For this review, take the finished solid that the model builds, in its own axes (mm). Round coordinates to 2 decimals unless told otherwise and drop trailing zeros. Order: outer loops, then holes, each group sorted by start corner. A loop starts at its lowest first (then second) coordinate and runs counter-clockwise, first axis right, second up. Notation, with made-up numbers: (68, -33.75) - (78, -33.75) arc R20 ccw to (78, -25.75) - close; hole circle Ø10 at (21.25, 70). An arc over 180 degrees is marked (long way). One line per item, written item: value.
Autodesk Inventor part; units mm, degrees
ref_plane "YZ Plane" through (0, 0, 0) normal (1, 0, 0) x (0, 1, 0)
ref_plane "XZ Plane" through (0, 0, 0) normal (0, 1, 0) x (-1, 0, 0)
ref_plane "XY Plane" through (0, 0, 0) normal (0, 0, 1) x (1, 0, 0)
sketch "Sketch1" plane through (0, 0, 0) normal (1, 0, 0) x (0, 1, 0)
  line L0 (3.175, 0) -> (-3.175, 0) construction
  line L1 (3.175, 1.5875) -> (-3.175, 1.5875) construction
  line L2 (-3.175, -1.5875) -> (3.175, -1.5875) construction
  arc A0 (3.175, -1.5875) -> (3.175, 1.5875) centre (3.175, 0) ccw construction
  arc A1 (-3.175, 1.5875) -> (-3.175, -1.5875) centre (-3.175, 0) ccw construction
  circle A2 centre (3.175, -12.7) radius 1.7526
  circle A3 centre (-3.175, -7.9375) radius 1.7526
  line L3 (3.175, -1.8415) -> (-3.175, -1.8415)
  arc A4 (-3.175, 1.8415) -> (-3.175, -1.8415) centre (-3.175, 0) ccw
  line L4 (-3.175, 1.8415) -> (3.175, 1.8415)
  arc A5 (3.175, -1.8415) -> (3.175, 1.8415) centre (3.175, 0) ccw
  arc A6 (1.27, -15.24) -> (6.35, -12.7) centre (3.175, -12.7) ccw
  arc A7 (-6.35, -7.9375) -> (-5.08, -10.4775) centre (-3.175, -7.9375) ccw
  line L5 (-5.08, -10.4775) -> (1.27, -15.24)
  line L6 (6.35, -12.7) -> (6.35, 0)
  line L7 (-6.35, -7.9375) -> (-6.35, 0)
  circle A8 centre (3.175, 12.7) radius 1.7526
  circle A9 centre (-3.175, 7.9375) radius 1.7526
  arc A10 (6.35, 12.7) -> (1.27, 15.24) centre (3.175, 12.7) ccw
  arc A11 (-5.08, 10.4775) -> (-6.35, 7.9375) centre (-3.175, 7.9375) ccw
  line L8 (-5.08, 10.4775) -> (1.27, 15.24)
  line L9 (6.35, 12.7) -> (6.35, 0)
  line L10 (-6.35, 7.9375) -> (-6.35, 0)
  point P0 (0, 0)
  dimension "d0" = 3.175
  dimension "d1" = 3.175
  dimension "d4" = 3.5052
  dimension "d5" = 12.7
  dimension "d6" = 3.175
  dimension "d7" = 3.5052
  dimension "d8" = 3.175
  dimension "d9" = 4.7625
  dimension "d10" = 0.254
  dimension "d11" = 6.35
  dimension "d12" = 6.35
extrude "Extrusion1" add sketch "Sketch1" along normal blind 1.5875
properties part number "Pin Cap - Slot" material "Aluminum 6061"
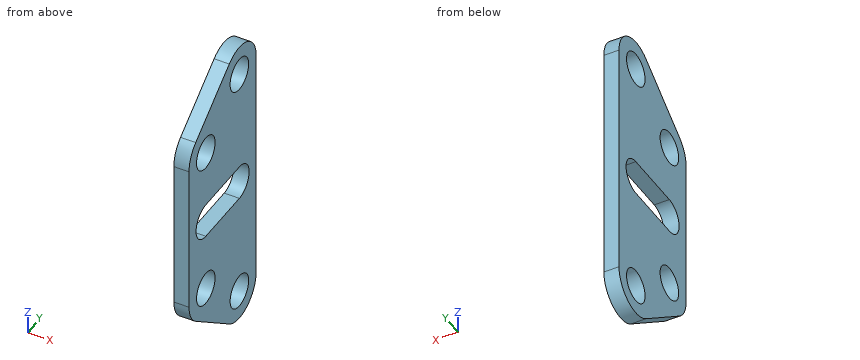
Item 1: Take a section at A-A (x = 0.85). Count the separate pieces of the cut face and the enclosed holes in it, plus the area to 3 significant figures.
Returned:
separate pieces: 1
enclosed holes: 5
area: 272 mm^2
Item 2: Take a section at D-D (z = 10). Write out the cut boundary in (x, y).
Returned:
outline: (0, -5.59) - (1.59, -5.59) - (1.59, 6.35) - (0, 6.35) - close
Item 3: For P1, Ø0.8, axis at x = 0.5, y = -1, coming from the +Z side; P2, Ø0.8, axis at x = 1, y = -0.5, coming from the -Z side, all flat-tipped, find the tip position at first contact; note any pin that passes through.
Returned:
P1: z = 13.84
P2: z = -14.21
Item 4: Take a section at C-C (y = 0.5). Write out the cut boundary in (x, z).
Returned:
outline: (0, -14.66) - (1.59, -14.66) - (1.59, -1.84) - (0, -1.84) - close; (0, 1.84) - (1.59, 1.84) - (1.59, 14.66) - (0, 14.66) - close
Item 5: Take a section at B-B (z = 0). Write out the cut boundary in (x, y).
Returned:
outline: (0, -6.35) - (1.59, -6.35) - (1.59, -5.02) - (0, -5.02) - close; (0, 5.02) - (1.59, 5.02) - (1.59, 6.35) - (0, 6.35) - close
Item 6: Wall thickness on line 1 (Z direction, x = 0.3, y = 4.75); line 2 (Z direction, x = 1, y = 4.25); line 3 (Z direction, x = 0.3, y = -0.25): over which ranges is each line inside the solid? List them lowest first.
Returned:
line 1: -15.46 to -13.47, -11.93 to -0.95, 0.95 to 11.93, 13.47 to 15.46
line 2: -15.69 to -14.08, -11.32 to -1.5, 1.5 to 11.32, 14.08 to 15.69
line 3: -14.1 to -1.84, 1.84 to 14.1
